Source: CAD feature listing. Evaluate the final solid. Frame: model axes, mm. A direction names the side the tool comes from. Coordinates: 2 decimals unless noted, no trailing zeros. Write each loop counter-clockwise with the first axis right and the second up, starting at its lowest first coordinate (ties: lowest second). Pieces come first, ordered by that corner, then holes. Notation, with made-up numbers: (8.5, 1.25) - (21.5, 1.25) arc R9 cw to (21.5, 5.25) - close; hole circle Ø1 at (79.25, -4.75). An arc over 180 degrees is marked (long way). One line per question, with ' | ' between items. Start each with the question number.
Q1. Cut plane C-C, the plane z = 0. Return loops of the section in (x, y).
Q2. Cut plane D-D, the plane y = 3.25. Return loops of the section in (x, z), plus the area to 3 significant figures.
Q3. Contact query for flat-ended pins moving along their axis: P1, Ø6.5, axis at x = 47.8, z = -27.8, coming from the +Y side; P2, Ø3, axis at x = 26.11, z = -30, coming from the +Y side; P3, Ø10, axis at y = 22, z = -3, coming from the +X side; P4, Ø4, axis at y = 16, z = -21, coming from the +X side. Output: stop coordinate, or through.
Q4. Access query for faces 1 (the face through (-37.5, 4.93, 0.16)), 2 (the face through (31.113, 19.86, -29.89)), 3 (the face through (55, 5, 0)). Directions: +Z, -Z, +X, -X, +Y, -Y. A direction counts if a zero-diameter tool reaches every point of the face in a straight line with its end or side. Return the directions, or none.
Q5. Line query: line 1 (Z direction, x = -32, y = 26); line 2 (Z direction, x = -7, y = 8.25); line 3 (X direction, y = 18.5, z = 30). Output: solid intervals per line, ascending.
Q6. Cut plane A-A, the plane x = -8. Return loops of the section in (y, z), plus the area to 3 significant figures.
Q7. Cut plane B-B, the plane y = 20. Return loops of the section in (x, z).
Q8. Draft query along X for faces 4 (the face through (31.113, 19.86, 30.11)), 5 (the face through (-50.28, 15.21, 28.13)), 6 (the face through (-9, 15, -35)). Return one class per face: +X half, -X half, draft (parallel to the pull), parting line (faces both ways), or undercut.
```python
from build123d import *

# Parameters (mm, degrees)
SKETCH1_R           = 2.5
BOSS_EXTRUDE1_DEPTH = 10
SKETCH1_6_R         = 5
BOSS_EXTRUDE2_DEPTH = 30
SKETCH3_R           = 2.5
CUT_EXTRUDE1_DEPTH  = 30
SKETCH6_R           = 2.6
CUT_EXTRUDE3_DEPTH  = 11


with BuildPart() as part:
    # Sketch1 → Boss-Extrude1 (new body)
    with BuildSketch(Plane(origin=(0, 0, 0), x_dir=(1, 0, 0), z_dir=(0, 1, 0))):
        with BuildLine():
            Line((-45, -35), (45, -35))
            ThreePointArc((45, -35), (52.071067812, -32.071067812), (55, -25))
            Line((55, -25), (55, 25))
            ThreePointArc((55, 25), (52.071067812, 32.071067812), (45, 35))
            Line((45, 35), (-45, 35))
            ThreePointArc((-45, 35), (-52.071067812, 32.071067812), (-55, 25))
            Line((-55, 25), (-55, -25))
            ThreePointArc((-55, -25), (-52.071067812, -32.071067812), (-45, -35))
        make_face()
        with Locations(Location((47.803300859, -27.803300859, 0), (0, 0, 270))):
            Circle(SKETCH1_R, mode=Mode.SUBTRACT)
        with BuildLine():
            Line((-30, 7.5), (30, 7.5))
            ThreePointArc((30, 7.5), (37.5, 0), (30, -7.5))
            Line((30, -7.5), (-30, -7.5))
            ThreePointArc((-30, -7.5), (-37.5, 0), (-30, 7.5))
        make_face(mode=Mode.SUBTRACT)
        with Locations(Location((47.803300859, 27.803300859, 0), (0, 0, 270))):
            Circle(SKETCH1_R, mode=Mode.SUBTRACT)
    extrude(amount=BOSS_EXTRUDE1_DEPTH)

    # Sketch1_6 → Boss-Extrude2 (add)
    with BuildSketch(Plane(origin=(0, 0, 0), x_dir=(1, 0, 0), z_dir=(0, 1, 0))):
        with BuildLine():
            Line((26.113792714, 35), (-45, 35))
            ThreePointArc((-45, 35), (-52.071067812, 32.071067812), (-55, 25))
            Line((-55, 25), (-55, -25))
            ThreePointArc((-55, -25), (-52.071067812, -32.071067812), (-45, -35))
            Line((-45, -35), (26.113792684, -35))
            ThreePointArc((26.113792684, -35), (21.113792714, -29.999999992), (26.1137927, -25))
            Line((26.1137927, -25), (-40, -25))
            ThreePointArc((-40, -25), (-43.535533906, -23.535533906), (-45, -20))
            Line((-45, -20), (-45, 20))
            ThreePointArc((-45, 20), (-43.535533906, 23.535533906), (-40, 25))
            Line((-40, 25), (26.113792714, 25))
            ThreePointArc((26.113792714, 25), (21.113792714, 30), (26.113792714, 35))
        make_face()
        with Locations((26.113792714, 30)):
            Circle(SKETCH1_6_R)
        with Locations((26.113792714, -30)):
            Circle(SKETCH1_6_R)
    extrude(amount=BOSS_EXTRUDE2_DEPTH)

    # Sketch3 → Cut-Extrude1 (cut)
    with BuildSketch(Plane(origin=(0, 30, 0), x_dir=(1, 0, 0), z_dir=(0, 1, 0))):
        with Locations(Location((-47.803300859, 27.803300859, 0), (0, 0, 270))):
            Circle(SKETCH3_R)
        with Locations(Location((-47.803300859, -27.803300859, 0), (0, 0, 90))):
            Circle(SKETCH3_R)
        with Locations(Location((26.113792714, 30, 0), (0, 0, 270))):
            Circle(SKETCH3_R)
        with Locations(Location((26.113792714, -30, 0), (0, 0, 90))):
            Circle(SKETCH3_R)
    extrude(amount=-CUT_EXTRUDE1_DEPTH, mode=Mode.SUBTRACT)

    # Sketch6 → Cut-Extrude3 (cut)
    with BuildSketch(Plane(origin=(-45, 0, 0), x_dir=(0, 0, -1), z_dir=(1, 0, 0))):
        with Locations((0, 20)):
            Circle(SKETCH6_R)
    extrude(amount=-CUT_EXTRUDE3_DEPTH, mode=Mode.SUBTRACT)


solid = part.part
```
Reply:
1) outline: (-55, 0) - (-37.5, 0) - (-37.5, 10) - (-45, 10) - (-45, 17.4) - (-55, 17.4) - close; (-55, 22.6) - (-45, 22.6) - (-45, 30) - (-55, 30) - close; (37.5, 0) - (55, 0) - (55, 10) - (37.5, 10) - close
2) outline: (-55, -25) arc R10 ccw to (-45, -35) - (45, -35) arc R10 ccw to (55, -25) - (55, 25) arc R10 ccw to (45, 35) - (-45, 35) arc R10 ccw to (-55, 25) - close; hole circle Ø5 at (-47.8, -27.8); hole circle Ø5 at (-47.8, 27.8); hole (-30, -7.5) - (30, -7.5) arc R7.5 ccw to (30, 7.5) - (-30, 7.5) arc R7.5 ccw to start; hole circle Ø5 at (26.11, -30); hole circle Ø5 at (26.11, 30); hole circle Ø5 at (47.8, -27.8); hole circle Ø5 at (47.8, 27.8) | area: 6,420 mm^2
3) P1: stops at y = 10 | P2: passes through | P3: stops at x = -45 | P4: stops at x = -44
4) face 1: +Y, -Y | face 2: +X, +Y | face 3: +Z, -Z, +X, +Y, -Y
5) line 1: z = -35 to -25, 25 to 35 | line 2: z = -35 to -7.5, 7.5 to 35 | line 3: x = -53.66 to -49, -46.61 to 23.61, 28.61 to 31.11
6) outline: (0, -35) - (30, -35) - (30, -25) - (10, -25) - (10, -7.5) - (0, -7.5) - close; (0, 7.5) - (10, 7.5) - (10, 25) - (30, 25) - (30, 35) - (0, 35) - close | area: 950 mm^2
7) outline: (-55, -25) arc R10 ccw to (-45, -35) - (26.11, -35) arc R5 ccw to (26.11, -25) - (-40, -25) arc R5 cw to (-45, -20) - (-45, -2.6) - (-55, -2.6) - close; (-55, 2.6) - (-45, 2.6) - (-45, 20) arc R5 cw to (-40, 25) - (26.11, 25) arc R5 ccw to (26.11, 35) - (-45, 35) arc R10 ccw to (-55, 25) - close; hole circle Ø5 at (-47.8, -27.8); hole circle Ø5 at (-47.8, 27.8); hole circle Ø5 at (26.11, -30); hole circle Ø5 at (26.11, 30)
8) face 4: +X half | face 5: undercut | face 6: draft
